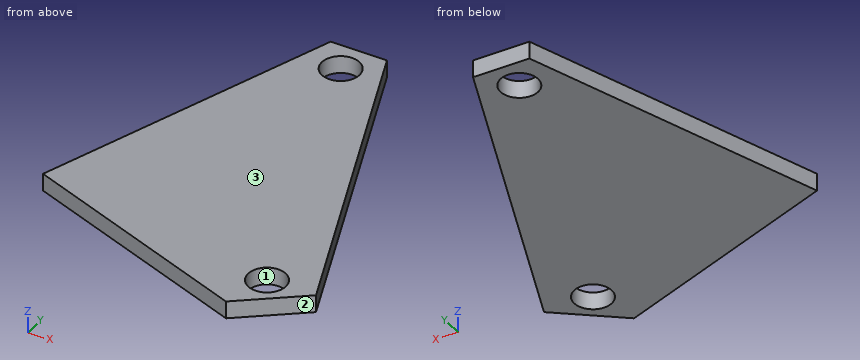
```python
from build123d import *

# Parameters (mm, degrees)
SKETCH1_R           = 3.429
BOSS_EXTRUDE1_DEPTH = 3.175


with BuildPart() as part:
    # Sketch1 → Boss-Extrude1 (new body)
    with BuildSketch(Plane.XY.offset(117.785358826)):
        Polygon((54.178453288, 19.606929499), (42.949199141, 11.069173633), (0.699486381, 27.001944289), (21.019486381, 80.885489203), (31.179486381, 80.885489203), align=None)
        with Locations((45.489199141, 19.381944289)):
            Circle(SKETCH1_R, mode=Mode.SUBTRACT)
        with Locations((26.099486381, 75.297489203)):
            Circle(SKETCH1_R, mode=Mode.SUBTRACT)
    extrude(amount=BOSS_EXTRUDE1_DEPTH)


solid = part.part
```
For this review, take the finished solid that the model builds, in its own axes (mm). Face numbers are marked on the shaded views. Round coordinates to 2 decimals unless told otherwise and drop trailing zeros. Write each loop counter-clockwise with the first axis right and the second up, starting at its lowest first coordinate (ties: lowest second). Pieces come first, ordered by that corner, then holes. Notation, with made-up numbers: (72, 69.25) -> (76, 69.25) arc R30 cw to (76, 98.25) -> close; hole circle Ø2 at (50.5, -34). An arc over 180 degrees is marked (long way). Use one line per item in the form item = value.
Q1. The part is to be moulded in two halves that separate along Y. For the marked faces 1, 2 and 3, say which applies: released by +Y, released by -Y, zero draft, split by the parting line, or undercut.
Resolved:
face_1 = undercut
face_2 = released by -Y
face_3 = zero draft
Q2. Clearance check with a flat-ended pin moving along its axis: pin 1 Ø9 at (x, y) = (26.1, 75.3) entering from +Z. State where the tip first meets the part, or that it passes through.
Resolved:
pin_1 = 120.96
Q3. Consider section D-D (y = 61). State the section outline as (x, z) points.
Resolved:
outline = (13.52, 117.79) -> (38.64, 117.79) -> (38.64, 120.96) -> (13.52, 120.96) -> close
Q4. Consider section B-B (z = 120.1). State the section outline as (x, y) points, then the cut area to 3 significant figures.
Resolved:
outline = (0.7, 27) -> (42.95, 11.07) -> (54.18, 19.61) -> (31.18, 80.89) -> (21.02, 80.89) -> close; hole circle Ø6.86 at (26.1, 75.3); hole circle Ø6.86 at (45.49, 19.38)
area = 2,020 mm²
Q5. To check wall thickness, follow probe 1 along Y at (x, z) = (30, 120.6); probe 2 along X at (y, z) = (70, 120.55); probe 3 along Y at (x, z) = (25.5, 119.8). State the ranges of each line that lie inside material, in increasing order. Write a range as from..to.
Resolved:
probe_1 = 15.95..80.89
probe_2 = 16.91..35.27
probe_3 = 17.65..71.92, 78.67..80.89
Q6. Consider section C-C (x = 24). State the section outline as (y, z) points, then the cut area to 3 significant figures.
Resolved:
outline = (18.22, 117.79) -> (72.59, 117.79) -> (72.59, 120.96) -> (18.22, 120.96) -> close; (78.01, 117.79) -> (80.89, 117.79) -> (80.89, 120.96) -> (78.01, 120.96) -> close
area = 182 mm²
Q7. Consider section A-A (x = 48). State the section outline as (y, z) points, then the cut area to 3 significant figures.
Resolved:
outline = (14.91, 117.79) -> (17.05, 117.79) -> (17.05, 120.96) -> (14.91, 120.96) -> close; (21.72, 117.79) -> (36.07, 117.79) -> (36.07, 120.96) -> (21.72, 120.96) -> close
area = 52.4 mm²
